Drawing for the job (mm, zero at the part's lowest x, y, z). A direction names the side the tool comes from. Coordinates: 2 decimals unless noted, no trailing zeros. Write each loop counter-clockwise with the first axis right and the second up, starting at its lowest first coordinate (ties: lowest second). Pieces come first, ordered by that corner, then holes. Notation, with made-up numbers: (44, 79) - (85, 79) arc R19 cw to (85, 111) - close; hole circle Ø1 at (34.25, -24). An arc over 180 degrees is marked (long way). Write each question's results on one line, items separated by ' | '.
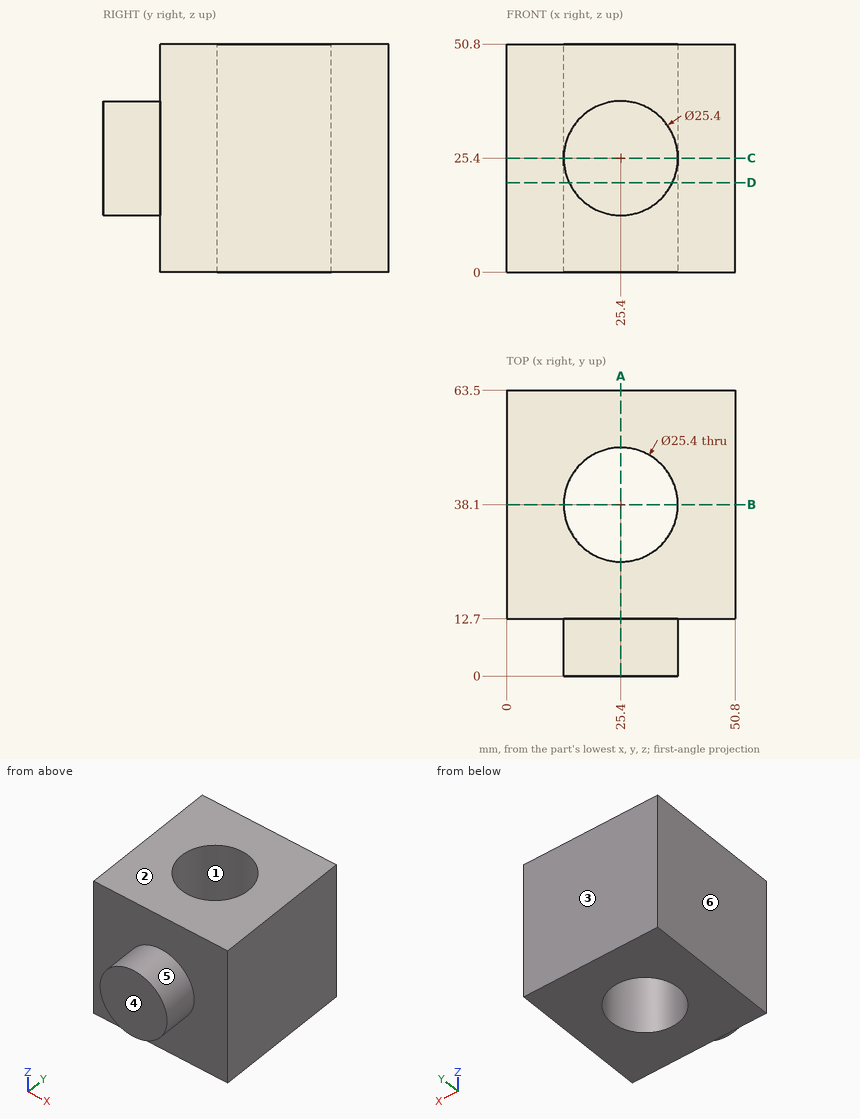
(1) Saw through at A-A on x = 25.4. Write the cut outline in (y, z).
Return value:
outline: (0, 12.7) - (12.7, 12.7) - (12.7, 0) - (25.4, 0) - (25.4, 50.8) - (12.7, 50.8) - (12.7, 38.1) - (0, 38.1) - close; (50.8, 0) - (63.5, 0) - (63.5, 50.8) - (50.8, 50.8) - close
(2) Two-plate mould, pull along Y, no slides. Class the marked faces 1, 2, 3 and 4: released by +Y, released by -Y, zero draft, split by the parting line, or undercut.
Return value:
face 1: undercut | face 2: zero draft | face 3: released by +Y | face 4: released by -Y
(3) Saw through at B-B on y = 38.1. Write the cut outline in (x, z), then the cut area to 3 significant figures.
Return value:
outline: (0, 0) - (12.7, 0) - (12.7, 50.8) - (0, 50.8) - close; (38.1, 0) - (50.8, 0) - (50.8, 50.8) - (38.1, 50.8) - close | area: 1,290 mm^2
(4) Wall check: line 1 (Y direction, x = 25.4, z = 26); line 2 (Y direction, x = 47, z = 14); line 3 (X direction, y = 38, z = 21). Give the ranges that are in metal, low to high. Write a range as from..to.
Return value:
line 1: y = 0..25.4, 50.8..63.5 | line 2: y = 12.7..63.5 | line 3: x = 0..12.7, 38.1..50.8
(5) Flat gauge pins, fed straight in: P1, Ø2, axis at x = 21.5, z = 41, coming from the -Y side; P2, Ø1.5, axis at x = 39, y = 9, coming from the +Z side. Where does each tip first touch, or does it go through?
Return value:
P1: stops at y = 12.7 | P2: passes through
(6) Saw through at C-C on z = 25.4. Write the cut outline in (x, y), then the cut area to 3 significant figures.
Return value:
outline: (0, 12.7) - (12.7, 12.7) - (12.7, 0) - (38.1, 0) - (38.1, 12.7) - (50.8, 12.7) - (50.8, 63.5) - (0, 63.5) - close; hole circle Ø25.4 at (25.4, 38.1) | area: 2,400 mm^2
(7) Saw through at D-D on z = 20. Write the cut outline in (x, y).
Return value:
outline: (0, 12.7) - (13.91, 12.7) - (13.91, 0) - (36.89, 0) - (36.89, 12.7) - (50.8, 12.7) - (50.8, 63.5) - (0, 63.5) - close; hole circle Ø25.4 at (25.4, 38.1)
(8) 3-axis set-ups, long thin cutter, end or side, ignore diameter. For the marked faces 5 and 6: which of +Z, -Z, +X, -X, +Y, -Y reach the whole face in a straight line?
Return value:
face 5: -Y | face 6: +Z, -Z, -X, +Y, -Y
